Autodesk Inventor part; units mm, degrees
ref_plane "YZ Plane" through (0, 0, 0) normal (1, 0, 0) x (0, 1, 0)
ref_plane "XZ Plane" through (0, 0, 0) normal (0, 1, 0) x (-1, 0, 0)
ref_plane "XY Plane" through (0, 0, 0) normal (0, 0, 1) x (1, 0, 0)
sketch "Эскиз1" plane through (0, 0, 0) normal (0, 0, 1) x (1, 0, 0)
  line L0 (1, 18) -> (1, 2)
  line L1 (1, 2) -> (17, 2)
  line L2 (17, 2) -> (17, 18)
  line L3 (17, 18) -> (1, 18)
  line L4 (1, -2) -> (1, -18)
  line L5 (1, -18) -> (17, -18)
  line L6 (17, -18) -> (17, -2)
  line L7 (17, -2) -> (1, -2)
  line L8 (-22.5, -9) -> (-22.5, -29.5)
  arc A0 (-22.5, -29.5) -> (-19.5, -32.5) centre (-19.5, -29.5) ccw
  line L9 (-19.5, -32.5) -> (19.5, -32.5)
  arc A1 (19.5, -32.5) -> (22.5, -29.5) centre (19.5, -29.5) ccw
  line L10 (22.5, -29.5) -> (22.5, 29.5)
  arc A2 (22.5, 29.5) -> (19.5, 32.5) centre (19.5, 29.5) ccw
  line L11 (19.5, 32.5) -> (-19.5, 32.5)
  arc A3 (-19.5, 32.5) -> (-22.5, 29.5) centre (-19.5, 29.5) ccw
  line L12 (-22.5, 29.5) -> (-22.5, 9)
  line L13 (-22.5, 9) -> (-2, 9)
  line L14 (-2, 9) -> (-2, -9)
  line L15 (-2, -9) -> (-22.5, -9)
  line L16 (1, 18) -> (17, 18)
  line L17 (17, 18) -> (17, 2)
  line L18 (17, 2) -> (1, 2)
  line L19 (1, 2) -> (1, 18)
  line L20 (1, -2) -> (17, -2)
  line L21 (17, -2) -> (17, -18)
  line L22 (17, -18) -> (1, -18)
  line L23 (1, -18) -> (1, -2)
  circle A4 centre (-18, 28) radius 1.5
  circle A5 centre (18, 28) radius 1.5
  circle A6 centre (18, -28) radius 1.5
  circle A7 centre (-18, -28) radius 1.5
  line L24 (-22.5, 9) -> (-22.5, -9)
  point P0 (0, 0)
extrude "Выдавливание1" add sketch "Эскиз1" along normal blind 1
properties part number "level3_up"
Source: CAD feature listing. Evaluate the final solid. Frame: model axes, mm. Give positions to 0.01 mm unless a question says otherwise; leave off trailing zeros. Order: outer loops, then holes, each group sorted by start corner. A loop starts at its lowest first (then second) coordinate and runs counter-clockwise, first axis right, second up. Notation, with made-up numbers: (-27.75, -30) -> (-17.75, -30) arc R29 ccw to (-17.75, -2) -> close; hole circle Ø9 at (49.25, -24.75). An arc over 180 degrees is marked (long way). Use a Markdown table: item, result.
Q1. Pull-direction query (Y, two-part tool) for faces 1 (the face through (0, 0, 1)), 2 (the face through (-21.6, -31.64, 0.49)), 3 (the face through (-19.11, -29.01, 0.49)); classes: +Y half, -Y half, draft (parallel to the pull), parting line (faces both ways), or undercut.
A:
| item | result |
|---|---|
| face 1 | draft |
| face 2 | -Y half |
| face 3 | undercut |
Q2. Section A-A (x = -18). Return the cut outline in (y, z).
A:
| item | result |
|---|---|
| outline | (-32.5, 0) -> (-29.5, 0) -> (-29.5, 1) -> (-32.5, 1) -> close; (-26.5, 0) -> (26.5, 0) -> (26.5, 1) -> (-26.5, 1) -> close; (29.5, 0) -> (32.5, 0) -> (32.5, 1) -> (29.5, 1) -> close |
Q3. Section D-D (z = 0.55). Return the cut outline in (x, y), and give its area (3 significant figures).
A:
| item | result |
|---|---|
| outline | (-22.5, -29.5) arc R3 ccw to (-19.5, -32.5) -> (19.5, -32.5) arc R3 ccw to (22.5, -29.5) -> (22.5, 29.5) arc R3 ccw to (19.5, 32.5) -> (-19.5, 32.5) arc R3 ccw to (-22.5, 29.5) -> close; hole circle Ø3 at (-18, -28); hole circle Ø3 at (-18, 28); hole (1, -18) -> (17, -18) -> (17, -2) -> (1, -2) -> close; hole (1, 2) -> (17, 2) -> (17, 18) -> (1, 18) -> close; hole circle Ø3 at (18, -28); hole circle Ø3 at (18, 28) |
| area | 2,380 mm^2 |
Q4. Section B-B (y = -8.5). Return the cut outline in (x, z).
A:
| item | result |
|---|---|
| outline | (-22.5, 0) -> (1, 0) -> (1, 1) -> (-22.5, 1) -> close; (17, 0) -> (22.5, 0) -> (22.5, 1) -> (17, 1) -> close |
Q5. Section C-C (y = -28). Return the cut outline in (x, z), and give its area (3 significant figures).
A:
| item | result |
|---|---|
| outline | (-22.5, 0) -> (-19.5, 0) -> (-19.5, 1) -> (-22.5, 1) -> close; (-16.5, 0) -> (16.5, 0) -> (16.5, 1) -> (-16.5, 1) -> close; (19.5, 0) -> (22.5, 0) -> (22.5, 1) -> (19.5, 1) -> close |
| area | 39.0 mm^2 |
Q6. Material intervals for line 1 (Y direction, x = 18, z = 0.5); line 2 (Y direction, x = 6, z = 0.1); line 3 (X direction, y = -6, z = 0.3), sorted ascending. Write a range as [from, to].
A:
| item | result |
|---|---|
| line 1 | [-32.5, -29.5], [-26.5, 26.5], [29.5, 32.5] |
| line 2 | [-32.5, -18], [-2, 2], [18, 32.5] |
| line 3 | [-22.5, 1], [17, 22.5] |
